```python
from build123d import *

# Parameters (mm, degrees)
SKETCH1_W          = 101.6
SKETCH1_H          = 50.8
REVOLVE1_ANGLE     = 72
SKETCH2_W          = 101.6
SKETCH2_H          = 50.8
CUT_EXTRUDE1_DEPTH = 0.635
SKETCH3_W          = 100.932321488
SKETCH3_H          = 50.8
CUT_EXTRUDE2_DEPTH = 0.635
CUT_EXTRUDE3_REACH = 151.001


with BuildPart() as part:
    # Sketch1 → Revolve1 (revolve)
    with BuildSketch(Plane.XY):
        with Locations((-50.8, 25.4)):
            Rectangle(SKETCH1_W, SKETCH1_H)
    revolve(axis=Axis((0, 0, 0), (0, 1, 0)), revolution_arc=REVOLVE1_ANGLE)

    # Sketch2 → Cut-Extrude1 (cut)
    with BuildSketch(Plane(origin=(0, 0, 0), x_dir=(0.3090169943749449, 0, -0.9510565162951544), z_dir=(0.9510565162951544, 0, 0.3090169943749449))):
        with Locations((-50.8, 25.4)):
            Rectangle(SKETCH2_W, SKETCH2_H)
    extrude(amount=-CUT_EXTRUDE1_DEPTH, mode=Mode.SUBTRACT)

    # Sketch3 → Cut-Extrude2 (cut)
    with BuildSketch(Plane(origin=(0, 0, 0), x_dir=(-1, 0, 0), z_dir=(0, 0, -1))):
        with Locations((51.133839256, 25.4)):
            Rectangle(SKETCH3_W, SKETCH3_H)
    extrude(amount=-CUT_EXTRUDE2_DEPTH, mode=Mode.SUBTRACT)

    # Sketch4 → Cut-Extrude3 (cut, up to next)
    with BuildSketch(Plane(origin=(0, 50.8, 0), x_dir=(1, 0, 0), z_dir=(0, 1, 0)), mode=Mode.PRIVATE) as cut_extrude3_sk1:
        Polygon((-1.116550937, -1.38148727), (-1.658905685, -0.635), (-0.874002519, -0.635), align=None)
    cut_extrude3_tool1 = extrude(cut_extrude3_sk1.sketch, amount=-CUT_EXTRUDE3_REACH, mode=Mode.PRIVATE) & part.part
    add(cut_extrude3_tool1.solids().sort_by_distance((-1.216486, 50.8, 0.883829))[0], mode=Mode.SUBTRACT)


solid = part.part
```
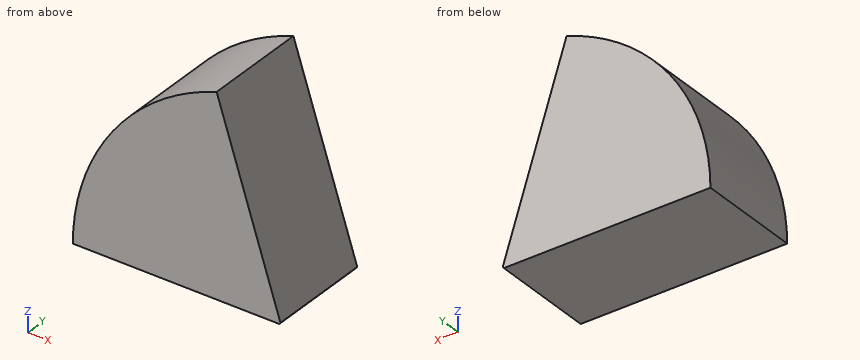
The model under review builds one solid part; all positions refer to its coordinate system, in mm. Give positions to 0.01 mm unless a question says otherwise; leave off trailing zeros. Write each loop counter-clockwise with the first axis right and the second up, starting at its lowest first coordinate (ties: lowest second). Pieces come first, ordered by that corner, then holes. Notation, with made-up numbers: (-6.75, 70.25) - (20.25, 70.25) arc R19 cw to (20.25, 103.25) - close; hole circle Ø3 at (71.25, -11). An arc over 180 degrees is marked (long way). Answer in a Markdown table with one row per item. Add a question column.
1. We need section A-A on y = 42.5. Write out the cut boundary in (x, z) (3 decimals), then the cut area to 3 significant figures.
2. Wall thickness on line 1 along Z through (x, y) = (-69, 36.5) (3 decimals); line 2 along X through (y, z) = (26, 92.5); line 3 along X through (y, z) = (10, 8): over which ranges is each line inside the solid? List them lowest first. Write a range as [from, to].
3. We need section B-B on z = 65. Write out the cut boundary in (x, y), then the cut area to 3 significant figures.
4. Insertion check: P1, Ø5, axis at x = -85, y = 14.5, coming from the +Z side; P2, Ø3, axis at y = 20.5, z = 19.5, coming from the +X side; P3, Ø5, axis at x = -45, y = 36.5, coming from the +Z side. Each pin has a flat end and moves straight along its axis. Give the tip position at first contact, or say it passes through.
Ans:
| question | item | result |
|---|---|---|
| 1 | outline | (-101.598, 0.635) - (-1.659, 0.635) - (-1.117, 1.381) - (-31.999, 96.429) arc R101.6 ccw to start |
| 1 | area | 6,360 mm^2 |
| 2 | line 1 | z = [0.635, 74.576] |
| 2 | line 2 | x = [-42.03, -30.72] |
| 2 | line 3 | x = [-101.28, -3.27] |
| 3 | outline | (-78.09, 0) - (-21.79, 0) - (-21.79, 50.8) - (-78.09, 50.8) - close |
| 3 | area | 2,860 mm^2 |
| 4 | P1 | stops at z = 59.3 |
| 4 | P2 | stops at x = -6.52 |
| 4 | P3 | stops at z = 92.28 |
